The figure shows three views and two pictorial views of one solid part (mm, origin at its lowest corner). Answer the questions. A direction names the side the tool comes from. Round coordinates to 2 decimals unless told otherwise and drop trailing zeros. Write each loop counter-clockwise with the first axis right and the second up, starting at its lowest first coordinate (ties: lowest second). Pieces come first, ordered by that corner, then holes.
Item 1: Find section B-B on x = 6.5. Give the vertices of the cut face in (y, z).
Item 2: For a pull along X with two mould halves and no side action, classify the marked faces 1, 2 and 3 as +X half, -X half, draft (parallel to the pull), parting line (faces both ways), or undercut.
Item 3: Find the intervals of material crossed by probe 1 along Y at (x, z) = (37, 1); probe 2 along Y at (x, z) = (47.5, 10.75); probe 3 along Z at (x, y) = (27, 23.25), in increasing order.
Item 4: Each of these flat-tipped pins is pushed along its axis until it touches: pin 1 (11 mm diameter, centred on x = 37.3, y = 12.7, fed in from -Z); pin 2 (5 mm diameter, centred on x = 27, y = 12.7, fed in from +Z); pin 3 (2.5 mm diameter, centred on x = 47.5, y = 12.7, fed in from +Z); pin 4 (9 mm diameter, centred on x = 27, y = 12.7, fed in from +Z). Where does it stop, or does it pass through?
Item 5: Find section C-C on y = 23.5. Give the vertices of the cut face in (x, z).
Item 6: Find section A-A on z = 13.25. Give the vertices of the cut face in (x, y).
Item 7: A tool of negligible diameter and unlimited length cuts with its end or side. For the marked faces 4, 5 and 6, from which of +Z, -Z, +X, -X, +Y, -Y can it reach the whole face along a straight path? Write none if from no direction.
Item 8: Find section D-D on z = 6.75. Give the vertices of the cut face in (x, y), then the cut area to 3 significant figures.
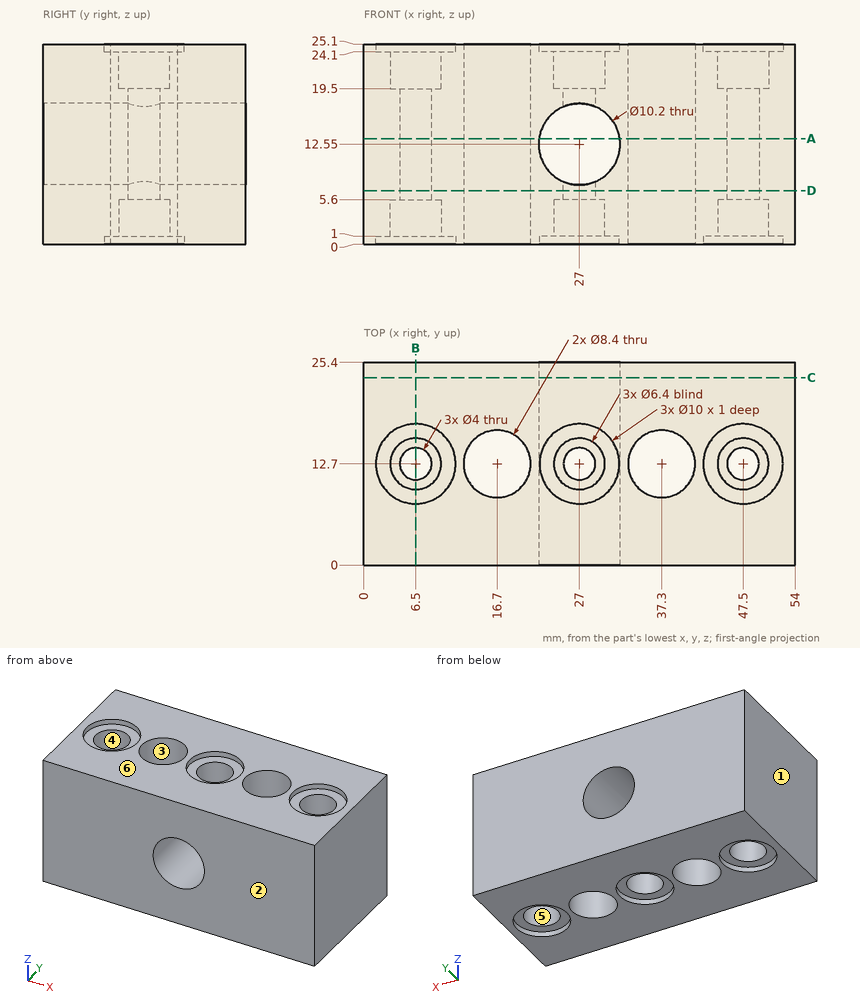
Check values:
1. outline: (0, 0) - (7.7, 0) - (7.7, 1) - (9.5, 1) - (9.5, 5.6) - (10.7, 5.6) - (10.7, 19.5) - (9.5, 19.5) - (9.5, 24.1) - (7.7, 24.1) - (7.7, 25.1) - (0, 25.1) - close; (14.7, 5.6) - (15.9, 5.6) - (15.9, 1) - (17.7, 1) - (17.7, 0) - (25.4, 0) - (25.4, 25.1) - (17.7, 25.1) - (17.7, 24.1) - (15.9, 24.1) - (15.9, 19.5) - (14.7, 19.5) - close
2. face 1: -X half
2. face 2: draft
2. face 3: undercut
3. probe 1: y = 0 to 8.51, 16.89 to 25.4
3. probe 2: y = 0 to 10.7, 14.7 to 25.4
3. probe 3: z = 0 to 7.45, 17.65 to 25.1
4. pin 1: stops at z = 0
4. pin 2: stops at z = 19.5
4. pin 3: passes through
4. pin 4: stops at z = 24.1
5. outline: (0, 0) - (54, 0) - (54, 25.1) - (0, 25.1) - close; hole circle Ø10.2 at (27, 12.55)
6. outline: (0, 0) - (21.95, 0) - (21.95, 25.4) - (0, 25.4) - close; (32.05, 0) - (54, 0) - (54, 25.4) - (32.05, 25.4) - close; hole circle Ø4 at (6.5, 12.7); hole circle Ø8.4 at (16.7, 12.7); hole circle Ø8.4 at (37.3, 12.7); hole circle Ø4 at (47.5, 12.7)
7. face 4: +Z
7. face 5: -Z
7. face 6: +Z, +X, -X, +Y, -Y
8. outline: (0, 0) - (54, 0) - (54, 25.4) - (0, 25.4) - close; hole circle Ø4 at (6.5, 12.7); hole circle Ø8.4 at (16.7, 12.7); hole circle Ø4 at (27, 12.7); hole circle Ø8.4 at (37.3, 12.7); hole circle Ø4 at (47.5, 12.7)
8. area: 1,220 mm2
